Job drawing, mm, ordinate dimensions from the low corner. One solid piece. A direction names the side the tool comes from. Give positions to 0.01 mm unless a question says otherwise; leave off trailing zeros. Order: outer loops, then holes, each group sorted by start corner. A loop starts at its lowest first (then second) coordinate and runs counter-clockwise, first axis right, second up.
Item 1: Band-saw the part on B-B on y = 18.5. Give the cut face in (x, z), plus the area to 3 significant figures.
Item 2: Band-saw the part on A-A on z = 5.5. Give the cut face in (x, y), plus the area to 3 significant figures.
Item 3: Two-plate mould, pull along X, no slides. Class the marked faces 3, 4 and 5: released by +X, released by -X, zero draft, split by the parting line, or undercut.
Item 4: Wall check: L1, parallel to Y at x = 87.5, z = 5.75; L2, parallel to X at y = 17.5, z = 7.25; L3, parallel to X at y = 9.5, z = 3.5. Give the ranges that are in metal, low to high.
Item 5: Which spindle directions (+Z, -Z, +X, -X, +Y, -Y) get a long thin tool onto all of the face, cutting with end or side? Do the marked faces 1 and 2. Say none if no direction does.
Item 6: Band-saw the part on D-D on y = 11.5. Give the cut face in (x, z).
Item 7: Flat gauge pin, fed straight in: P1, Ø6, axis at x = 59, y = 11, coming from the +Z side. Where does the tip first touch, or does it go through?
Item 8: Band-saw the part on C-C on x = 18.5. Give the cut face in (y, z).
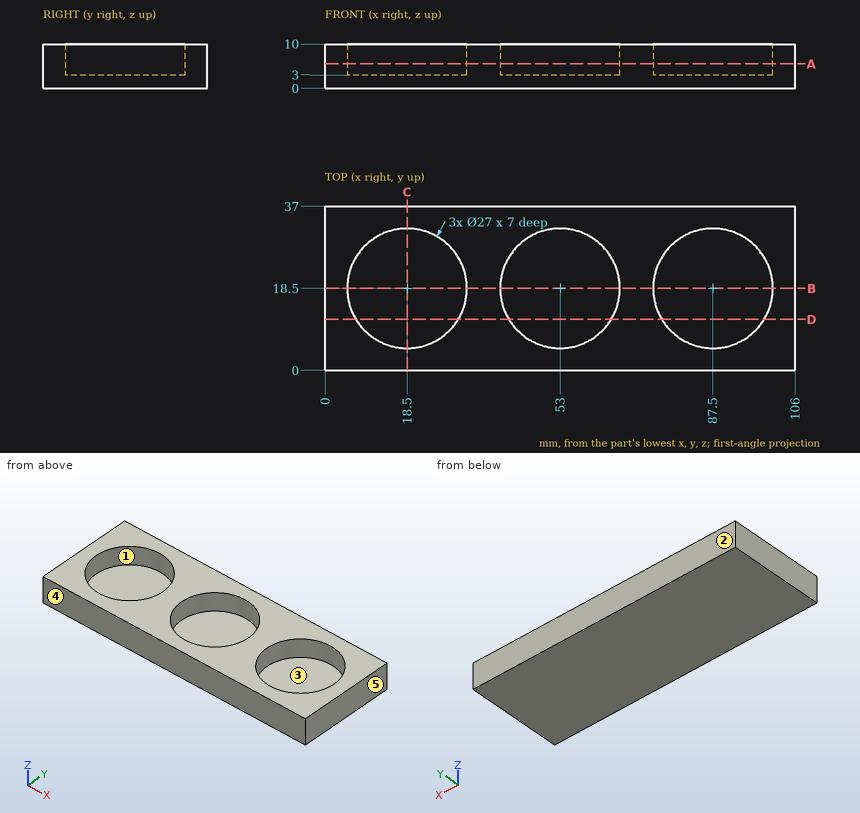
The answers:
1. outline: (0, 0) - (106, 0) - (106, 10) - (101, 10) - (101, 3) - (74, 3) - (74, 10) - (66.5, 10) - (66.5, 3) - (39.5, 3) - (39.5, 10) - (32, 10) - (32, 3) - (5, 3) - (5, 10) - (0, 10) - close
1. area: 493 mm2
2. outline: (0, 0) - (106, 0) - (106, 37) - (0, 37) - close; hole circle Ø27 at (18.5, 18.5); hole circle Ø27 at (53, 18.5); hole circle Ø27 at (87.5, 18.5)
2. area: 2,200 mm2
3. face 3: undercut
3. face 4: zero draft
3. face 5: released by +X
4. L1: y = 0 to 5, 32 to 37
4. L2: x = 0 to 5.04, 31.96 to 39.54, 66.46 to 74.04, 100.96 to 106
4. L3: x = 0 to 8.44, 28.56 to 42.94, 63.06 to 77.44, 97.56 to 106
5. face 1: +Z
5. face 2: +Z, -Z, +X, -X, +Y
6. outline: (0, 0) - (106, 0) - (106, 10) - (99.04, 10) - (99.04, 3) - (75.96, 3) - (75.96, 10) - (64.54, 10) - (64.54, 3) - (41.46, 3) - (41.46, 10) - (30.04, 10) - (30.04, 3) - (6.96, 3) - (6.96, 10) - (0, 10) - close
7. P1: stops at z = 3
8. outline: (0, 0) - (37, 0) - (37, 10) - (32, 10) - (32, 3) - (5, 3) - (5, 10) - (0, 10) - close
